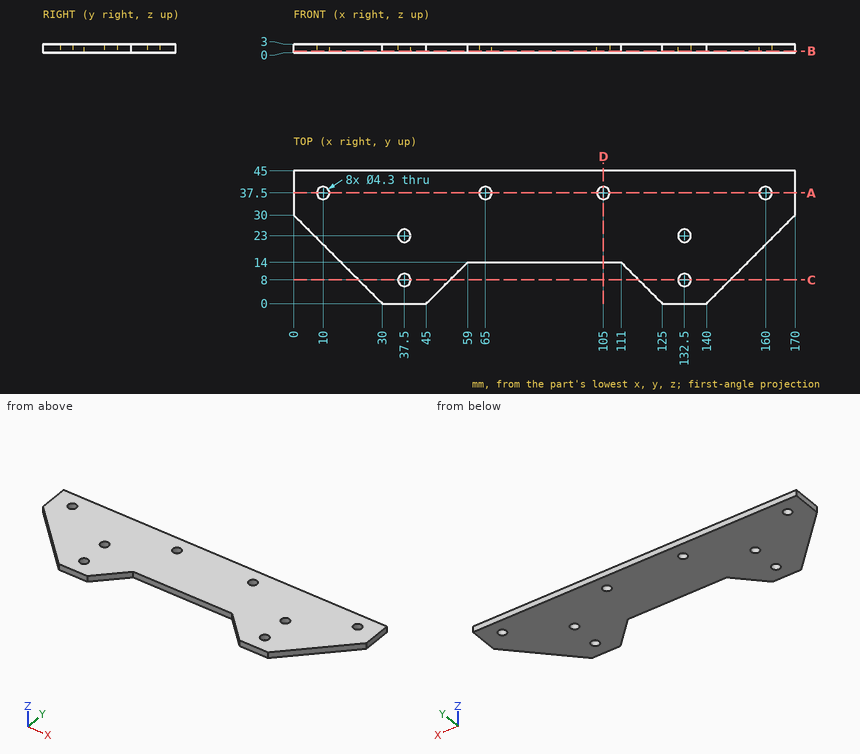
Source: three-view drawing plus pictorial views. Frame: mm from the lowest corner of the part. Give positions to 0.01 mm unless a question says otherwise; leave off trailing zeros. Loops run counter-clockwise (first coordinate to the right, second up) from the corner with the lowest first, then second, coordinate; pieces in that order, holes last. Notation, with made-up numbers: M 63.5,20.25 L 116.5,20.25 A8 cw 116.5,25.25 Z; hole C 74,67.5 d5. An arc over 180 degrees is marked long. Put each result on its own line as item: value.
Q1. Section C-C (y = 8). Return the cut outline in (x, z).
Response values:
outline: M 22,0 L 35.35,0 L 35.35,3 L 22,3 Z; M 39.65,0 L 53,0 L 53,3 L 39.65,3 Z; M 117,0 L 130.35,0 L 130.35,3 L 117,3 Z; M 134.65,0 L 148,0 L 148,3 L 134.65,3 Z
Q2. Pin query (flat end, axial travel): P1, Ø1.5, axis at x = 144, z = 2, coming from the -Y side. Return the tip coordinate at first contact, or that it passes through.
Response values:
P1: stops at y = 3.25
Q3. Section D-D (x = 105). Return the cut outline in (y, z), and give its area (3 significant figures).
Response values:
outline: M 14,0 L 35.35,0 L 35.35,3 L 14,3 Z; M 39.65,0 L 45,0 L 45,3 L 39.65,3 Z
area: 80.1 mm²
Q4. Section B-B (z = 0.55). Count the separate pieces of the cut face and the enclosed holes in it, and give its area (3 significant figures).
Response values:
separate pieces: 1
enclosed holes: 8
area: 5,710 mm²
Q5. Line query: probe 1 along Y at (x, z) = (132.5, 1.4); probe 2 along X at (y, z) = (37.5, 2.05); probe 3 along Y at (x, z) = (105, 2). Output: solid intervals per line, ascending. Write a range as [from, to].
Response values:
probe 1: y = [0, 5.85], [10.15, 20.85], [25.15, 45]
probe 2: x = [0, 7.85], [12.15, 62.85], [67.15, 102.85], [107.15, 157.85], [162.15, 170]
probe 3: y = [14, 35.35], [39.65, 45]
Q6. Section A-A (y = 37.5). Return the cut outline in (x, z).
Response values:
outline: M 0,0 L 7.85,0 L 7.85,3 L 0,3 Z; M 12.15,0 L 62.85,0 L 62.85,3 L 12.15,3 Z; M 67.15,0 L 102.85,0 L 102.85,3 L 67.15,3 Z; M 107.15,0 L 157.85,0 L 157.85,3 L 107.15,3 Z; M 162.15,0 L 170,0 L 170,3 L 162.15,3 Z
